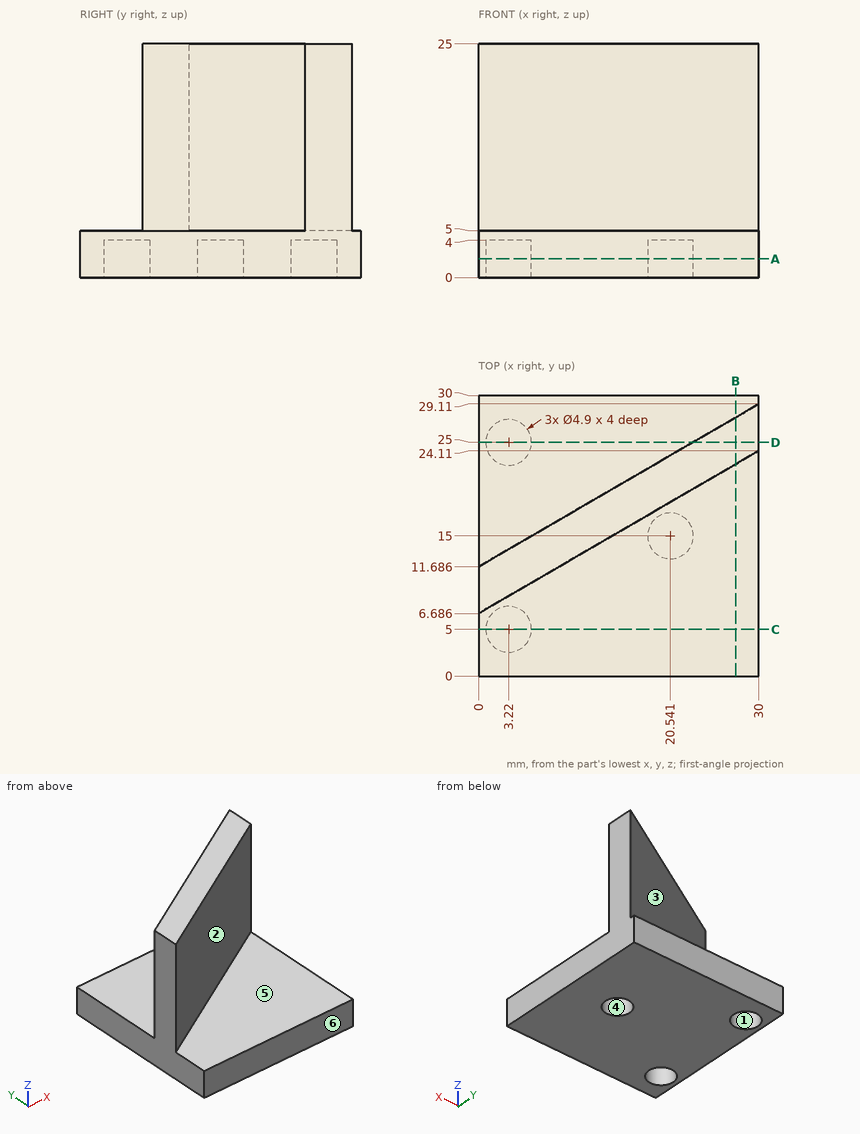
The figure shows three views and two pictorial views of one solid part (mm, origin at its lowest corner). Answer the questions. A direction names the side the tool comes from. Coordinates: 2 decimals unless noted, no trailing zeros. Loops run counter-clockwise (first coordinate to the right, second up) from the corner with the lowest first, then second, coordinate; pieces in that order, holes last. Notation, with made-up numbers: (39.25, 53) - (61.25, 53) arc R14 cw to (61.25, 58) - close; hole circle Ø4 at (-37.75, 63.25). An arc over 180 degrees is marked (long way). Write item = value, one per line.
1) Which of the six approach directions +Z, -Z, +X, -X, +Y, -Y give full straight-line access (tool end or side, diameter ignored) to the marked faces 1, 2 and 3?
Responses:
face_1 = -Z
face_2 = +Z, +X, -Y
face_3 = +Z, -X, +Y
2) Section D-D (y = 25) is taken. Determine the outline of the cut face in (x, z) (1 decimal), plus the area to 3 significant figures.
Responses:
outline = (0, 0) - (0.8, 0) - (0.8, 4) - (5.7, 4) - (5.7, 0) - (30, 0) - (30, 25) - (22.9, 25) - (22.9, 5) - (0, 5) - close
area = 272 mm^2
3) Determine the mould class of the marked faces 4, 5 and 6 for opening direction Y: pulls with the +Y half, pulls with the -Y half, needs draft (parallel to the pull), parting line crosses it, or undercut.
Responses:
face_4 = undercut
face_5 = needs draft
face_6 = pulls with the -Y half
4) Section A-A (z = 2) is taken. Determine the outline of the cut face in (x, y).
Responses:
outline = (0, 0) - (30, 0) - (30, 30) - (0, 30) - close; hole circle Ø4.9 at (3.22, 5); hole circle Ø4.9 at (3.22, 25); hole circle Ø4.9 at (20.54, 15)
5) Section C-C (y = 5) is taken. Determine the outline of the cut face in (x, z), plus the area to 3 significant figures.
Responses:
outline = (0, 0) - (0.77, 0) - (0.77, 4) - (5.67, 4) - (5.67, 0) - (30, 0) - (30, 5) - (0, 5) - close
area = 130 mm^2
6) Find the intervals of material crossed by line 1 along Y through (x, z) = (3.22, 2.4); line 2 along Z through (x, y) = (8.25, 4); line 3 along X through (y, z) = (27, 2) (1 decimal), in increasing order.
Responses:
line_1 = 0 to 2.55, 7.45 to 22.55, 27.45 to 30
line_2 = 0 to 5
line_3 = 0 to 1.8, 4.6 to 30
7) Each of these flat-tipped pins is pushed along its axis until it touches: P1, Ø3, axis at x = 23, z = 9.5, coming from the +Y side (1 decimal); P2, Ø7, axis at x = 22, y = 12.5, coming from the +Z side; P3, Ø2.5, axis at x = 4, y = 5.5, coming from the -Z side. Where does it stop, or does it pass through?
Responses:
P1 = 25.9
P2 = 5
P3 = 4
8) Section B-B (x = 27.5) is taken. Determine the outline of the cut face in (y, z), plus the area to 3 significant figures.
Responses:
outline = (0, 0) - (30, 0) - (30, 5) - (27.66, 5) - (27.66, 25) - (22.66, 25) - (22.66, 5) - (0, 5) - close
area = 250 mm^2
